Autodesk Inventor part; units mm, degrees
ref_plane "YZ Plane" through (0, 0, 0) normal (1, 0, 0) x (0, 1, 0)
ref_plane "XZ Plane" through (0, 0, 0) normal (0, 1, 0) x (-1, 0, 0)
ref_plane "XY Plane" through (0, 0, 0) normal (0, 0, 1) x (1, 0, 0)
sketch "Sketch1" plane through (0, 0, 0) normal (0, 1, 0) x (-1, 0, 0)
  line L0 (53.975, 21.59) -> (-53.975, 21.59)
  line L1 (-53.975, 21.59) -> (-53.975, -21.59)
  line L2 (-53.975, -21.59) -> (53.975, -21.59)
  line L3 (53.975, -21.59) -> (53.975, 21.59)
  line L4 (53.975, 21.59) -> (-53.975, -21.59) construction
  line L5 (-53.975, 21.59) -> (53.975, -21.59) construction
  line L6 (60.325, 27.94) -> (-60.325, 27.94)
  line L7 (-60.325, 27.94) -> (-60.325, -27.94)
  line L8 (-60.325, -27.94) -> (60.325, -27.94)
  line L9 (60.325, -27.94) -> (60.325, 27.94)
  line L10 (60.325, 27.94) -> (-60.325, -27.94) construction
  line L11 (-60.325, 27.94) -> (60.325, -27.94) construction
  point P0 (0, 0)
  dimension "d0" = 43.18
  dimension "d1" = 107.95
  dimension "d2" = 6.35
  dimension "d3" = 6.35
extrude "Extrusion1" add sketch "Sketch1" against normal blind 12.065 contours L3 L2 L1 L0 | L9 L8 L7 L6
extrude "Extrusion2" add sketch "Sketch1" along normal blind 8.89
sketch "Sketch2" plane through (0, 0, 0) normal (0, 1, 0) x (1, 0, 0)
  line L0 (-53.975, 21.59) -> (-53.975, -21.59) construction
  line L1 (-53.975, 0) -> (53.975, 0) construction
  line L2 (53.975, -21.59) -> (53.975, 21.59) construction
  point P0 (0, 0)
  point P1 (-41.275, 0)
  point P2 (41.275, 0)
  dimension "d8" = 12.7
  dimension "d9" = 12.7
hole "Hole1" at (-41.275, 0, 0) at (41.275, 0, 0) direction (0, -1, 0) diameter 5.1054 end through all counterbore diameter 10.16 counterbore depth 2.54
sketch "Sketch5" plane through (0, -12.065, 0) normal (0, -1, 0) x (1, 0, 0)
  line L0 (-25.4, -27.94) -> (25.4, -27.94)
  line L1 (25.4, -27.94) -> (25.4, 27.94)
  line L2 (25.4, 27.94) -> (-25.4, 27.94)
  line L3 (-25.4, 27.94) -> (-25.4, -27.94)
  line L4 (-25.4, -27.94) -> (25.4, 27.94) construction
  line L5 (25.4, -27.94) -> (-25.4, 27.94) construction
  point P0 (0, 0)
  dimension "d27" = 50.8
  dimension "d28" = 55.88
extrude "Extrusion6" add sketch "Sketch5" along normal blind 19.05
sketch "Sketch11" plane through (-60.325, 8.89, 27.94) normal (0, 0, 1) x (1, 0, 0)
  line L0 (0, -20.955) -> (0, 0) construction
  line L1 (0, -10.4775) -> (120.65, -10.4775) construction
  line L2 (120.65, 0) -> (120.65, -20.955) construction
  line L3 (52.9098, -4.1275) -> (48.5358, -16.8275)
  line L4 (48.5358, -16.8275) -> (46.7142, -16.8275)
  line L5 (46.7142, -16.8275) -> (42.3402, -4.1275)
  line L6 (42.3402, -4.1275) -> (44.1515, -4.1275)
  line L7 (44.1515, -4.1275) -> (47.6713, -14.6765)
  line L8 (47.6713, -14.6765) -> (51.1911, -4.1275)
  line L9 (51.1911, -4.1275) -> (52.9098, -4.1275)
  line L10 (58.56, -12.0418) -> (53.7537, -12.0418)
  line L11 (53.7537, -12.0418) -> (53.7537, -10.4981)
  line L12 (53.7537, -10.4981) -> (58.56, -10.4981)
  line L13 (58.56, -10.4981) -> (58.56, -12.0418)
  spline S0 degree 2 poles (68.1519, -10.4775) (68.1519, -13.8944) (66.1656, -17.0951) (64.0969, -17.0951) knots 0 0 0 1 2 2 2
  spline S1 degree 2 poles (64.0969, -17.0951) (61.9974, -17.0951) (60.0317, -13.8326) (60.0317, -10.4878) knots 0 0 0 1 2 2 2
  spline S2 degree 2 poles (60.0317, -10.4878) (60.0317, -7.0504) (62.018, -3.8702) (64.0969, -3.8702) knots 0 0 0 1 2 2 2
  spline S3 degree 2 poles (64.0969, -3.8702) (66.1861, -3.8702) (68.1519, -7.1636) (68.1519, -10.4775) knots 0 0 0 1 2 2 2
  spline S4 degree 2 poles (65.97, -14.3472) (66.217, -13.7194) (66.4229, -11.7846) (66.4229, -10.4775) knots 0 0 0 1 2 2 2
  spline S5 degree 2 poles (66.4229, -10.4775) (66.4229, -9.1704) (66.217, -7.2459) (65.9597, -6.5975) knots 0 0 0 1 2 2 2
  spline S6 degree 2 poles (65.9597, -6.5975) (65.7024, -5.9491) (64.8071, -5.2802) (64.0969, -5.2802) knots 0 0 0 1 2 2 2
  spline S7 degree 2 poles (64.0969, -5.2802) (63.3868, -5.2802) (62.4708, -5.9491) (62.2032, -6.6181) knots 0 0 0 1 2 2 2
  spline S8 degree 2 poles (62.2032, -6.6181) (61.9459, -7.2665) (61.7607, -9.2425) (61.7607, -10.4878) knots 0 0 0 1 2 2 2
  spline S9 degree 2 poles (61.7607, -10.4878) (61.7607, -11.8257) (61.9254, -13.6165) (62.193, -14.3163) knots 0 0 0 1 2 2 2
  spline S10 degree 2 poles (62.193, -14.3163) (62.44, -14.975) (63.3559, -15.6851) (64.0969, -15.6851) knots 0 0 0 1 2 2 2
  spline S11 degree 2 poles (64.0969, -15.6851) (64.7968, -15.6851) (65.7127, -15.0162) (65.97, -14.3472) knots 0 0 0 1 2 2 2
  line L14 (76.9719, -16.8275) -> (70.7763, -16.8275)
  line L15 (70.7763, -16.8275) -> (70.7763, -15.5307)
  line L16 (70.7763, -15.5307) -> (73.0816, -15.5307)
  line L17 (73.0816, -15.5307) -> (73.0816, -7.0195)
  line L18 (73.0816, -7.0195) -> (70.7763, -7.0195)
  line L19 (70.7763, -7.0195) -> (70.7763, -5.8565)
  spline S12 degree 2 poles (70.7763, -5.8565) (72.0833, -5.8565) (73.3183, -5.1155) (73.4006, -4.0863) knots 0 0 0 1 2 2 2
  line L20 (73.4006, -4.0863) -> (74.718, -4.0863)
  line L21 (74.718, -4.0863) -> (74.718, -15.5307)
  line L22 (74.718, -15.5307) -> (76.9719, -15.5307)
  line L23 (76.9719, -15.5307) -> (76.9719, -16.8275)
  point P0 (60.325, -8.89)
extrude "Extrusion8" cut sketch "Sketch11" against normal blind 2.54
sketch "Sketch12" plane through (-60.325, 8.89, 27.94) normal (0, 0, 1) x (1, 0, 0)
  line L0 (85.725, -40.005) -> (34.925, -40.005) construction
  line L1 (60.325, -40.005) -> (60.325, -0.5585) construction
  line L2 (63.9912, -40.005) -> (56.6588, -40.005)
  line L3 (56.6588, -40.005) -> (52.9927, -33.655)
  line L4 (52.9927, -33.655) -> (56.6588, -27.305)
  line L5 (56.6588, -27.305) -> (63.9912, -27.305)
  line L6 (63.9912, -27.305) -> (67.6573, -33.655)
  line L7 (67.6573, -33.655) -> (63.9912, -40.005)
  point P0 (60.325, -8.89)
  point P1 (60.325, -33.655)
  dimension "d86" = 12.7
extrude "Extrusion9" add sketch "Sketch12" along normal blind 60.96
mirror "Mirror5" about plane through (0, 0, 0) normal (0, 0, 1) of "Extrusion9"
equation "\"d0\" = innerWidth"
equation "\"d1\" = innerLength"
equation "\"d2\" = wallThickness"
equation "\"d3\" = wallThickness"
equation "\"d4\" = bottomThickness"
equation "\"d6\" = innerDepth"
equation "\"d27\" = lowerPostLength"
equation "\"d28\" = lowerPostWidth"
equation "\"d29\" = lowerPostHeight"
equation "\"d86\" = hexSize"
equation "\"innerWidth\" = 43.18"
equation "\"innerLength\" = 107.95"
equation "\"innerDepth\" = 8.89"
equation "\"wallThickness\" = 6.35"
equation "\"postDiameter\" = 9.525"
equation "\"holeCenterFromInnerWall\" = 12.7"
equation "\"bottomThickness\" = 12.065"
equation "\"d17\" = postDiameter"
equation "\"exteriorWidth\" = innerWidth + 2 * wallThickness"
equation "\"exteriorLength\" = innerLength + 2 * wallThickness"
equation "\"exteriorHeight\" = innerDepth + bottomThickness"
equation "\"d24\" = postDiameter"
equation "\"lowerPostWidth\" = exteriorWidth"
equation "\"lowerPostLength\" = 50.8"
equation "\"lowerPostCenterX\" = 0.5 * exteriorLength"
equation "\"lowerPostHeight\" = 19.05"
equation "\"lowerPostCenterY\" = postDiameter"
equation "\"setScrewCenters\" = 0.333333 * exteriorWidth"
equation "\"hexSize\" = 12.7"
properties part number "connectorToTubeBracketWithOffsetHexShaft-V01" material "PBT Plastic"
For this review, take the finished solid that the model builds, in its own axes (mm). A direction names the side the tool comes from. Give positions to 0.01 mm unless a question says otherwise; leave off trailing zeros. Write each loop counter-clockwise with the first axis right and the second up, starting at its lowest first coordinate (ties: lowest second). Pieces come first, ordered by that corner, then holes. Notation, with made-up numbers: M 36,-22.75 L 80,-22.75 A22 cw 80,14.25 Z; hole C 7.5,86 d11. An arc over 180 degrees is marked long. Answer as a JSON object with one key per item and string values. Group by question number.
Item 1: Tool access review of faces 4 (the flat face through (-46, -12.065, 0)), 5 (the flat face through (1, 0, 0)), 6 (the flat face through (5.525, -27.896, 57.993)), 7 (the flat face through (-11, -2, 25.4)): name each direction out of +Z, -Z, +X, -X, +Y, -Y from which nothing blocks a thin tool from reaching the whole face with its end or side.
Item 2: For probe 1 along X at (y, z) = (-1, 0) (3 decimals); probe 2 along X at (y, z) = (-6.5, 0) (3 decimals); probe 3 along Z at (x, y) = (23.5, 7.5), list the stretches that pass through material, from the lowest coordinate up. Write a range as [from, to].
Item 3: Consider section A-A on z = 0. Write out the cut boundary in (x, y) (3 decimals).
Item 4: Draft analysis for pull direction Y (two halves, no side actions). For faces 1 (the flat face through (6.4, -1.5, 25.4)), 2 (the flat face through (0, -18.415, -58)), 3 (the cylindrical face through (-36.768, -1.288, 2.344)), state which applies: +Y half, -Y half, draft (parallel to the pull), parting line (faces both ways), or undercut.
Item 5: Consider section C-C on z = -19. Write out the cut boundary in (x, y) (3 decimals), plus the area to 3 significant figures.
Item 6: For pin 1 Ø13 at (x, z) = (-41.275, 0) entering from +Y; pin 2 Ø8 at (y, z) = (-15.5, -14.5) entering from +X (3 decimals); pin 3 Ø17.5 at (x, z) = (39.5, -3) entering from -Y (3 decimals); pin 4 Ø2.5 at (x, y) = (18.5, 5) entering from -Z, all flat-tipped, find the tip position at first contact; note any pin that passes through.
Item 7: Consider section B-B on z = 73. Write out the cut boundary in (x, y) (3 decimals).
Check result:
{
 "1": {"face 4": "+Z, -Z, -X, -Y", "face 5": "+Y", "face 6": "+Z, +X, -Y", "face 7": "+Z"},
 "2": {"probe 1": "x = [-60.325, -46.355], [-36.195, 36.195], [46.355, 60.325]", "probe 2": "x = [-60.325, -43.828], [-38.722, 38.722], [43.828, 60.325]", "probe 3": "z = [-27.94, -21.59], [21.59, 27.94]"},
 "3": {"outline": "M -60.325,-12.065 L -43.828,-12.065 L -43.828,-2.54 L -46.355,-2.54 L -46.355,0 L -53.975,0 L -53.975,8.89 L -60.325,8.89 Z; M -38.722,-12.065 L -25.4,-12.065 L -25.4,-31.115 L 25.4,-31.115 L 25.4,-12.065 L 38.722,-12.065 L 38.722,-2.54 L 36.195,-2.54 L 36.195,0 L -36.195,0 L -36.195,-2.54 L -38.722,-2.54 Z; M 43.828,-12.065 L 60.325,-12.065 L 60.325,8.89 L 53.975,8.89 L 53.975,0 L 46.355,0 L 46.355,-2.54 L 43.828,-2.54 Z"},
 "4": {"face 1": "undercut", "face 2": "+Y half", "face 3": "draft"},
 "5": {"outline": "M -60.325,-12.065 L -25.4,-12.065 L -25.4,-31.115 L 25.4,-31.115 L 25.4,-12.065 L 60.325,-12.065 L 60.325,8.89 L 53.975,8.89 L 53.975,0 L -53.975,0 L -53.975,8.89 L -60.325,8.89 Z", "area": "2,540 mm^2"},
 "6": {"pin 1": "stops at y = 0", "pin 2": "stops at x = 60.325", "pin 3": "stops at y = -12.065", "pin 4": "stops at z = -27.94"},
 "7": {"outline": "M -7.332,-24.765 L -3.666,-31.115 L 3.666,-31.115 L 7.332,-24.765 L 3.666,-18.415 L -3.666,-18.415 Z"}
}
